Answer from the drawing. Dimensions are ordinates in mm from the lowest x, y and z of the part. A direction names the side the tool comes from. Coordinates: 2 decimals unless noted, no trailing zeros. Write each loop counter-clockwise with the first axis right and the second up, starting at its lowest first coordinate (ties: lowest second). Pieces come first, ordered by that corner, then holes.
(1) The part is cut by section A-A on x = 5.5. Determine the outline of the cut face in (y, z), plus the area to 3 significant figures.
(2) The part is cut by section C-C on x = 19. Determine the outline of the cut face in (y, z), plus the area to 3 significant figures.
(3) Straight lines are drawn through the part: line 1 (Y direction, x = 5.5, z = 17.45); line 2 (Z direction, x = 8.5, y = 18). For each, find the intervals that lie inside material, in ascending order.
(4) Given P1, Ø1.9, axis at x = 5.5, y = 32.5, coming from the +Z side; P2, Ø8, axis at y = 11.5, z = 9, coming from the -X side; P3, Ø3, axis at x = 32.5, y = 32.5, coming from the -Z side, each flat-ended and moving along its own axis, determine where each tip first touches the part or whether it passes through.
(5) Which of the six approach directions +Z, -Z, +X, -X, +Y, -Y give full straight-line access (tool end or side, diameter ignored) to the marked faces 1 and 2?
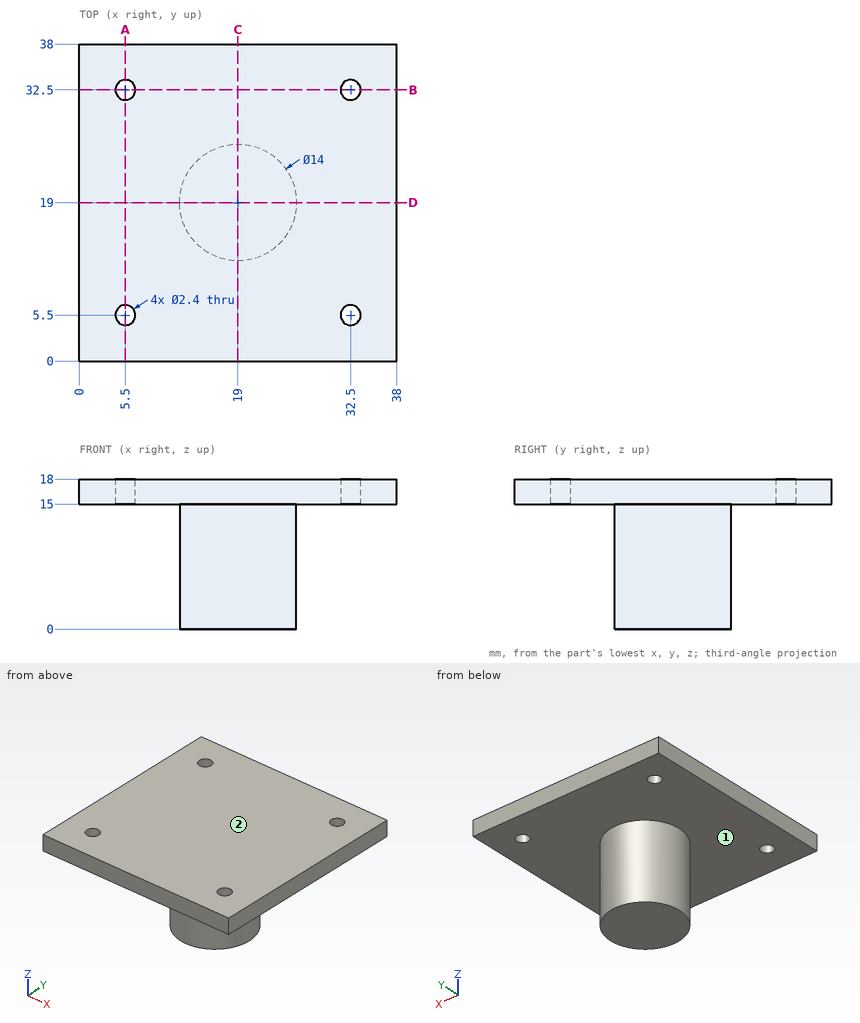
Model answer:
1. outline: (0, 15) - (4.3, 15) - (4.3, 18) - (0, 18) - close; (6.7, 15) - (31.3, 15) - (31.3, 18) - (6.7, 18) - close; (33.7, 15) - (38, 15) - (38, 18) - (33.7, 18) - close
1. area: 99.6 mm2
2. outline: (0, 15) - (12, 15) - (12, 0) - (26, 0) - (26, 15) - (38, 15) - (38, 18) - (0, 18) - close
2. area: 324 mm2
3. line 1: y = 0 to 4.3, 6.7 to 31.3, 33.7 to 38
3. line 2: z = 15 to 18
4. P1: passes through
4. P2: stops at x = 12.94
4. P3: stops at z = 15
5. face 1: -Z
5. face 2: +Z, +X, -X, +Y, -Y
